Geometry: see drawing. Coordinates: mm, zero at the bounding-box minimum. Round coordinates to 2 decimals unless told otherwise and drop trailing zeros. Order: outer loops, then holes, each group sorted by start corner. A loop starts at its lowest first (then second) coordinate and runs counter-clockwise, first axis right, second up. Notation, with made-up numbers: (18, 72.5) -> (37, 72.5) arc R30 ccw to (37, 111.5) -> close; hole circle Ø9 at (42.5, -25.5). An arc over 180 degrees is marked (long way). Answer as CSV lines item,"result". Start each with the question number.
(1) Line query: line 1 along X through (y, z) = (41.5, 45); line 2 along Z through (x, y) = (30, 11); line 3 along X through (y, z) = (27, 40.5). Output: solid intervals per line, ascending. Write a range as from..to.
(2) Section query C-C (y = 28). Output: boundary loops of the cut face in (x, z).
(3) Section query A-A (x = 30). Output: boundary loops of the cut face in (y, z).
(4) Section query B-B (z = 46). Output: boundary loops of the cut face in (x, y), plus the area to 3 significant figures.
(5) Contact query for a flat-ended pin moving along its axis: P1, Ø13, axis at x = 30, z = 46, coming from the -Y side. Output: stop coordinate, or through.
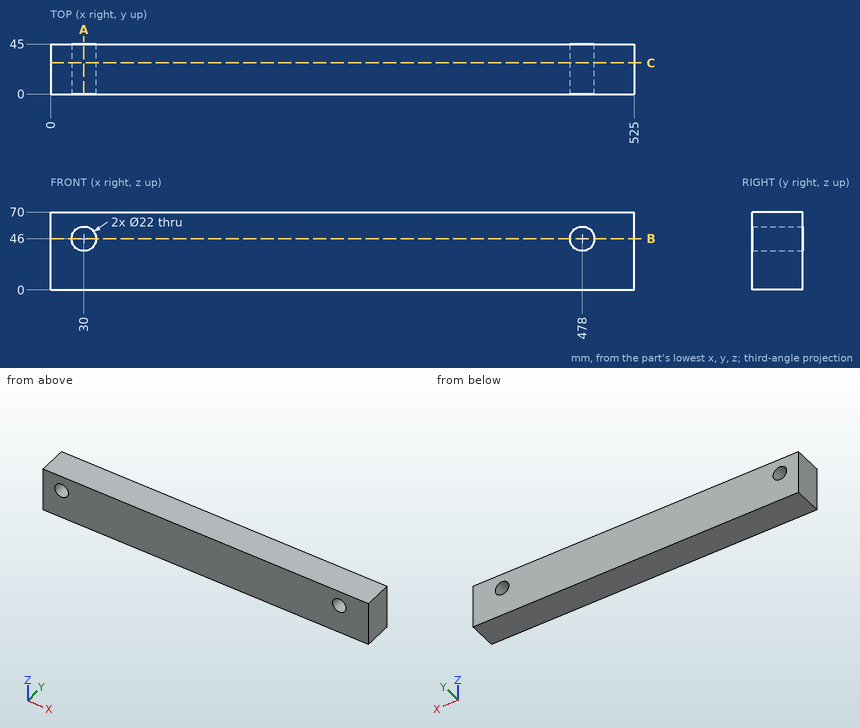
Answer block:
1,line 1,"0..19.05, 40.95..467.05, 488.95..525"
1,line 2,"0..35, 57..70"
1,line 3,"0..20.47, 39.53..468.47, 487.53..525"
2,outline,"(0, 0) -> (525, 0) -> (525, 70) -> (0, 70) -> close; hole circle Ø22 at (30, 46); hole circle Ø22 at (478, 46)"
3,outline,"(0, 0) -> (45, 0) -> (45, 35) -> (0, 35) -> close; (0, 57) -> (45, 57) -> (45, 70) -> (0, 70) -> close"
4,outline,"(0, 0) -> (19, 0) -> (19, 45) -> (0, 45) -> close; (41, 0) -> (467, 0) -> (467, 45) -> (41, 45) -> close; (489, 0) -> (525, 0) -> (525, 45) -> (489, 45) -> close"
4,area,"21,600 mm2"
5,P1,"through"
